For this review, take the finished solid that the model builds, in its own axes (mm). A direction names the side the tool comes from. Give positions to 0.01 mm unless a question says otherwise; leave off trailing zeros. Loops run counter-clockwise (first coordinate to the right, second up) from the corner with the lowest first, then second, coordinate; pieces in that order, holes last.
```python
from build123d import *

# Parameters (mm, degrees)
SZKIC1_W                        = 38.573617051
SZKIC1_H                        = 6
DODANIE_WYCI_GNI_CIE1_DEPTH     = 2
WYTNIJ_WYCI_GNI_CIE2_DEPTH      = 1
WYTNIJ_WYCI_GNI_CIE2_DEPTH_BACK = 38.075597401
SZKIC3_R                        = 1.6
DODANIE_WYCI_GNI_CIE2_DEPTH     = 1
SZKIC5_R                        = 1.6
WYTNIJ_WYCI_GNI_CIE3_DEPTH      = 38.142965991
ZAOKR_GLENIE1_R                 = 3


with BuildPart() as part:
    # Szkic1 → Dodanie-wyciągnięcie1 (new body)
    with BuildSketch(Plane.XY):
        with Locations((-15.012785421, 10.933333333)):
            Rectangle(SZKIC1_W, SZKIC1_H)
    extrude(amount=DODANIE_WYCI_GNI_CIE1_DEPTH)

    # Szkic3 → Wytnij-wyciągnięcie2 (cut, two sides: drawn at the far end of the back side and taken through both)
    with BuildSketch(Plane.XY.offset(2).offset(-WYTNIJ_WYCI_GNI_CIE2_DEPTH_BACK)):
        with Locations((-31.24872203, 10.943210033)):
            Circle(SZKIC3_R)
        with Locations((1.25127797, 10.943210033)):
            Circle(SZKIC3_R)
    extrude(amount=WYTNIJ_WYCI_GNI_CIE2_DEPTH + WYTNIJ_WYCI_GNI_CIE2_DEPTH_BACK, mode=Mode.SUBTRACT)

    # Szkic4 → Dodanie-wyciągnięcie2 (add)
    with BuildSketch(Plane.XY.offset(2)):
        Polygon((-34.299593946, 13.933333333), (-28.299593946, 13.933333333), (-28.299593946, 12.433333333), (-1.725976895, 12.433333333), (-1.725976895, 13.933333333), (4.274023105, 13.933333333), (4.274023105, 7.933333333), (-1.725976895, 7.933333333), (-1.725976895, 9.504700568), (-28.299593946, 9.504700568), (-28.299593946, 7.933333333), (-34.299593946, 7.933333333), align=None)
    extrude(amount=DODANIE_WYCI_GNI_CIE2_DEPTH)

    # Szkic5 → Wytnij-wyciągnięcie3 (cut, through all)
    with BuildSketch(Plane(origin=(0, 0, 0), x_dir=(-1, 0, 0), z_dir=(0, 0, -1))):
        with Locations((-1.25127797, 10.943210033)):
            Circle(SZKIC5_R)
        with Locations((31.24872203, 10.943210033)):
            Circle(SZKIC5_R)
    extrude(amount=-WYTNIJ_WYCI_GNI_CIE3_DEPTH, mode=Mode.SUBTRACT)

    # Zaokrąglenie1
    zaokr_glenie1_edges = [part.edges().sort_by_distance(p)[0] for p in [
        (-34.299593946, 7.933333333, 1.5),
        (-34.299593946, 13.933333333, 1.5),
        (4.274023105, 7.933333333, 1.5),
        (4.274023105, 13.933333333, 1.5),
    ]]
    fillet(zaokr_glenie1_edges, radius=ZAOKR_GLENIE1_R - 0.0001)  # a hair under: the kernel refuses the full size


solid = part.part
```
Item 1: Clearance check with flat-ended pins moving along their axes: pin 1 Ø0.5 at (x, y) = (-21, 9) entering from +Z; pin 2 Ø0.5 at (x, z) = (-19.5, 2.5) entering from +Y; pin 3 Ø1.1 at (y, z) = (13.5, 2.5) entering from +X. State where each tip first meets the part, or that it passes through.
Answer:
pin 1: stops at z = 2
pin 2: stops at y = 12.43
pin 3: stops at x = 3.5
Item 2: Take a section at C-C on y = 8.65. Give the boundary of the cut face in (x, z), and give its area (3 significant figures).
Answer:
outline: (-33.25, 0) - (3.22, 0) - (3.22, 3) - (-1.73, 3) - (-1.73, 2) - (-28.3, 2) - (-28.3, 3) - (-33.25, 3) - close
area: 82.8 mm2
Item 3: For L1, parallel to X at y = 12.3, z = 2.45; L2, parallel to X at y = 9.8, z = 2.4; L3, parallel to Z at x = -23.5, y = 8.8, list the stretches that pass through material, from the lowest coordinate up.
Answer:
L1: x = -33.97 to -32.1, -30.4 to 0.4, 2.1 to 3.94
L2: x = -34.08 to -32.37, -30.13 to 0.13, 2.37 to 4.05
L3: z = 0 to 2
Item 4: Take a section at A-A on x = -22.5. Give the boundary of the cut face in (y, z), and give its area (3 significant figures).
Answer:
outline: (7.93, 0) - (13.93, 0) - (13.93, 2) - (12.43, 2) - (12.43, 3) - (9.5, 3) - (9.5, 2) - (7.93, 2) - close
area: 14.9 mm2
Item 5: Take a section at B-B on y = 11.65. Give the boundary of the cut face in (x, z), and give its area (3 significant figures).
Answer:
outline: (-34.21, 0) - (-32.68, 0) - (-32.68, 3) - (-34.21, 3) - close; (-29.81, 0) - (-0.18, 0) - (-0.18, 3) - (-29.81, 3) - close; (2.69, 0) - (4.19, 0) - (4.19, 3) - (2.69, 3) - close
area: 98.0 mm2
Item 6: Tool access review of faces 4 (the cylindrical face through (-33.444, 8.835, 1.521)), 5 (the flat face through (-1.726, 8.7, 2.5)), 6 (the flat face through (-15, 13, 2)): name each direction out of +Z, -Z, +X, -X, +Y, -Y from which nothing blocks a thin tool from reaching the whole face with its end or side.
Answer:
face 4: +Z, -Z, -X, -Y
face 5: +Z, -Y
face 6: +Z, +Y
Item 7: The part is to be moulded in two halves that separate along X. For faces 1 (the flat face through (-15, 9, 2)), 2 (the cylindrical face through (-33.397, 13.078, 1.521)), 3 (the flat face through (-15, 11, 3)), say which applies: released by +X, released by -X, zero draft, split by the parting line, or undercut.
Answer:
face 1: undercut
face 2: released by -X
face 3: zero draft
